Check sheet for the modelled part. Datum: model origin and axes. Units: mm. Round coordinates to 2 decimals unless told otherwise and drop trailing zeros. Write each loop counter-clockwise with the first axis right and the second up, starting at its lowest first coordinate (ties: lowest second). Pieces come first, ordered by that corner, then holes.
Item 1: Material ranges on line 1 (Y direction, x = -6.5, z = 61); line 2 (Z direction, x = 1, y = 1068); line 3 (Z direction, x = -3, y = 994), recorded low to high.
Item 2: Cross-section at B-B on x = 0. Enter the section's corners in (y, z).
Item 3: Go/stop test with flat-tipped pins: pin 1 Ø8 at (x, y) = (-11.5, 660) entering from -Z; pin 2 Ø7.5 at (x, z) = (0, -39) entering from -Y; pin 3 Ø15.5 at (y, z) = (881.5, -32) entering from -X; pin 4 Ø12 at (x, z) = (13, 18) entering from -Y. Record where each tip stops, or that it passes through.
Item 4: Cross-section at C-C on y = 514. Enter the section's corners in (x, z), plus the area to 3 significant figures.
Item 5: Cross-section at A-A on z = 39. Enter the section's corners in (x, y).
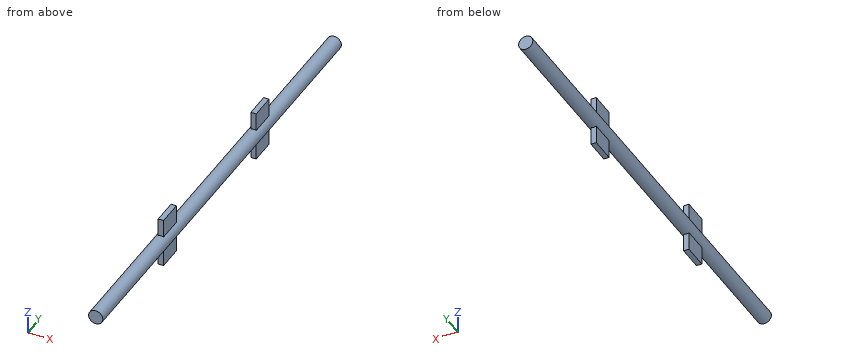
from build123d import *

# Parameters (mm, degrees)
ESQUISSE1_R        = 20
BOSS_EXTRU_1_DEPTH = 1300
ESQUISSE2_W        = 15
ESQUISSE2_H        = 70
BOSS_EXTRU_2_DEPTH = 70
ESQUISSE4_W        = 15
ESQUISSE4_H        = 70
BOSS_EXTRU_3_DEPTH = 70


with BuildPart() as part:
    # Esquisse1 → Boss.-Extru.1 (new body)
    with BuildSketch(Plane(origin=(0, 0, 0), x_dir=(1, 0, 0), z_dir=(0, 1, 0))):
        with Locations(Location((0, 0, 0), (0, 0, 270))):
            Circle(ESQUISSE1_R)
    extrude(amount=BOSS_EXTRU_1_DEPTH)

    # Esquisse2 → Boss.-Extru.2 (add, symmetric)
    with BuildSketch(Plane.XY):
        with Locations((0, 390)):
            Rectangle(ESQUISSE2_W, ESQUISSE2_H)
    extrude(amount=BOSS_EXTRU_2_DEPTH, both=True)

    # Esquisse4 → Boss.-Extru.3 (add, symmetric)
    with BuildSketch(Plane.XY):
        with Locations((0, 895)):
            Rectangle(ESQUISSE4_W, ESQUISSE4_H)
    extrude(amount=BOSS_EXTRU_3_DEPTH, both=True)


solid = part.part
Response values:
1. line 1: y = 355 to 425, 860 to 930
1. line 2: z = -19.97 to 19.97
1. line 3: z = -19.77 to 19.77
2. outline: (0, -20) - (355, -20) - (355, -70) - (425, -70) - (425, -20) - (860, -20) - (860, -70) - (930, -70) - (930, -20) - (1300, -20) - (1300, 20) - (930, 20) - (930, 70) - (860, 70) - (860, 20) - (425, 20) - (425, 70) - (355, 70) - (355, 20) - (0, 20) - close
3. pin 1: stops at z = -18.54
3. pin 2: stops at y = 355
3. pin 3: stops at x = -7.5
3. pin 4: stops at y = 0
4. outline: circle Ø40 at (0, 0)
4. area: 1,260 mm2
5. outline: (-7.5, 355) - (7.5, 355) - (7.5, 425) - (-7.5, 425) - close; (-7.5, 860) - (7.5, 860) - (7.5, 930) - (-7.5, 930) - close
